from build123d import *

# Parameters (mm, degrees)
SKETCH_1_W          = 83
SKETCH_1_H          = 53
SKETCH_1_W_2        = 80.2
SKETCH_1_H_2        = 50.2
EXTRUDE_1_DEPTH     = 35
SKETCH_3_W          = 80.2
SKETCH_3_H          = 50.2
EXTRUDE_2_DEPTH     = 1.4
SKETCH_4_W          = 5
SKETCH_4_H          = 5
SKETCH_4_R          = 0.95
EXTRUDE_3_DEPTH     = 12
SKETCH_5_W          = 41
SKETCH_5_H          = 7
CUT_EXTRUDE_1_DEPTH = 10
SKETCH_6_W          = 10
SKETCH_6_H          = 7
SKETCH_6_H_2        = 9
SKETCH_6_W_2        = 10.2
SKETCH_6_H_3        = 6
CUT_EXTRUDE_2_DEPTH = 10
SKETCH_8_W          = 21
SKETCH_8_H          = 21
CUT_EXTRUDE_4_DEPTH = 10
SKETCH_9_W          = 13
SKETCH_9_H          = 9.6
CUT_EXTRUDE_5_DEPTH = 10
FILLET_1_R          = 1
FILLET_2_R          = 1
SKETCH_11_W         = 17.500857193
SKETCH_11_H         = 7
CUT_EXTRUDE_7_DEPTH = 10
FILLET_5_R          = 1
SKETCH_13_R         = 6
CUT_EXTRUDE_8_DEPTH = 10
FILLET_6_R          = 1
FILLET_7_R          = 1


with BuildPart() as part:
    # 草图1 → 凸台-拉伸1 (new body)
    with BuildSketch(Plane(origin=(0, 0, 0), x_dir=(1, 0, 0), z_dir=(0, 1, 0))):
        with Locations((40.1, 25.1)):
            Rectangle(SKETCH_1_W, SKETCH_1_H)
        with Locations((40.1, 25.1)):
            Rectangle(SKETCH_1_W_2, SKETCH_1_H_2, mode=Mode.SUBTRACT)
    extrude(amount=EXTRUDE_1_DEPTH)

    # 草图3 → 凸台-拉伸2 (add)
    with BuildSketch(Plane(origin=(0, 0, 0), x_dir=(1, 0, 0), z_dir=(0, 1, 0))):
        with Locations((40.1, 25.1)):
            Rectangle(SKETCH_3_W, SKETCH_3_H)
    extrude(amount=EXTRUDE_2_DEPTH)

    # 草图4 → 凸台-拉伸3 (add)
    # profile 1 of 4: a face of its own
    with BuildSketch(Plane(origin=(0, 1.4, 0), x_dir=(1, 0, 0), z_dir=(0, 1, 0))):
        with Locations((2.5, 47.7)):
            Rectangle(SKETCH_4_W, SKETCH_4_H)
        with Locations(Location((2.5, 47.7, 0), (0, 0, 270))):
            Circle(SKETCH_4_R, mode=Mode.SUBTRACT)
    # profile 2 of 4: a face of its own
    with BuildSketch(Plane(origin=(0, 1.4, 0), x_dir=(1, 0, 0), z_dir=(0, 1, 0))):
        with Locations((2.5, 2.5)):
            Rectangle(SKETCH_4_W, SKETCH_4_H)
        with Locations(Location((2.5, 2.5, 0), (0, 0, 270))):
            Circle(SKETCH_4_R, mode=Mode.SUBTRACT)
    # profile 3 of 4: a face of its own
    with BuildSketch(Plane(origin=(0, 1.4, 0), x_dir=(1, 0, 0), z_dir=(0, 1, 0))):
        with Locations((77.7, 47.7)):
            Rectangle(SKETCH_4_W, SKETCH_4_H)
        with Locations(Location((77.7, 47.7, 0), (0, 0, 270))):
            Circle(SKETCH_4_R, mode=Mode.SUBTRACT)
    # profile 4 of 4: a face of its own
    with BuildSketch(Plane(origin=(0, 1.4, 0), x_dir=(1, 0, 0), z_dir=(0, 1, 0))):
        with Locations((77.7, 2.5)):
            Rectangle(SKETCH_4_W, SKETCH_4_H)
        with Locations(Location((77.7, 2.184711345, 0), (0, 0, 270))):
            Circle(SKETCH_4_R, mode=Mode.SUBTRACT)
    extrude(amount=EXTRUDE_3_DEPTH)

    # 草图5 → 切除-拉伸1 (cut)
    with BuildSketch(Plane.ZY.offset(-80.2)):
        with Locations((-25.5, 17.9)):
            Rectangle(SKETCH_5_W, SKETCH_5_H)
    extrude(amount=-CUT_EXTRUDE_1_DEPTH, mode=Mode.SUBTRACT)

    # 草图6 → 切除-拉伸2 (cut)
    with BuildSketch(Plane(origin=(0, 0, 0), x_dir=(0, 0, -1), z_dir=(1, 0, 0))):
        with Locations((10, 17.9)):
            Rectangle(SKETCH_6_W, SKETCH_6_H)
        with Locations((40.2, 20.9)):
            Rectangle(SKETCH_6_W, SKETCH_6_H_2)
        with Locations((25.1, 18.4)):
            Rectangle(SKETCH_6_W_2, SKETCH_6_H_3)
    extrude(amount=-CUT_EXTRUDE_2_DEPTH, mode=Mode.SUBTRACT)

    # 草图8 → 切除-拉伸4 (cut)
    with BuildSketch(Plane.XY.offset(-50.2)):
        with Locations((64.7, 24.9)):
            Rectangle(SKETCH_8_W, SKETCH_8_H)
    extrude(amount=-CUT_EXTRUDE_4_DEPTH, mode=Mode.SUBTRACT)

    # 草图9 → 切除-拉伸5 (cut)
    with BuildSketch(Plane(origin=(0, 0, 0), x_dir=(-1, 0, 0), z_dir=(0, 0, -1))):
        with Locations((-40.1, 30.2)):
            Rectangle(SKETCH_9_W, SKETCH_9_H)
    extrude(amount=-CUT_EXTRUDE_5_DEPTH, mode=Mode.SUBTRACT)

    # 圆角1
    fillet_1_edges = [part.edges().sort_by_distance(p)[0] for p in [
        (80.9, 21.4, -5),
        (80.9, 14.4, -5),
        (80.9, 14.4, -46),
        (80.9, 21.4, -46),
        (-0.7, 14.4, -5),
        (-0.7, 21.4, -5),
        (-0.7, 21.4, -15),
        (-0.7, 14.4, -15),
        (-0.7, 25.4, -45.2),
        (-0.7, 16.4, -45.2),
        (-0.7, 16.4, -35.2),
        (-0.7, 25.4, -35.2),
        (-0.7, 15.4, -20),
        (-0.7, 21.4, -20),
        (-0.7, 15.4, -30.2),
        (75.2, 14.4, -50.9),
        (54.2, 14.4, -50.9),
        (46.6, 25.4, 0.7),
        (33.6, 25.4, 0.7),
        (5, 7.4, -5),
        (5, 7.4, -45.2),
        (75.2, 7.4, -45.2),
        (75.2, 7.4, -5),
    ]]
    fillet(fillet_1_edges, radius=FILLET_1_R)

    # 圆角2
    fillet_2_edges = [part.edges().sort_by_distance(p)[0] for p in [
        (40.1, 0, -51.6),
        (81.6, 0, -25.1),
        (40.1, 0, 1.4),
        (-1.4, 0, -25.1),
        (-1.4, 17.5, -51.6),
        (81.6, 17.5, -51.6),
        (81.6, 17.5, 1.4),
        (-1.4, 17.5, 1.4),
    ]]
    fillet(fillet_2_edges, radius=FILLET_2_R)

    # 草图11 → 切除-拉伸7 (cut)
    with BuildSketch(Plane(origin=(0, 0, 0), x_dir=(-1, 0, 0), z_dir=(0, 0, -1))):
        with Locations((-61.449571404, 17.9)):
            Rectangle(SKETCH_11_W, SKETCH_11_H)
    extrude(amount=-CUT_EXTRUDE_7_DEPTH, mode=Mode.SUBTRACT)

    # 圆角5
    fillet_5_edges = [part.edges().sort_by_distance(p)[0] for p in [
        (70.2, 14.4, 0.7),
        (70.2, 21.4, 0.7),
        (52.699142807, 21.4, 0.7),
        (52.699142807, 14.4, 0.7),
    ]]
    fillet(fillet_5_edges, radius=FILLET_5_R)

    # 草图13 → 切除-拉伸8 (cut)
    with BuildSketch(Plane(origin=(0, 0, 0), x_dir=(0, 0, -1), z_dir=(1, 0, 0))):
        with Locations((35.2, 7.4)):
            Circle(SKETCH_13_R)
    extrude(amount=-CUT_EXTRUDE_8_DEPTH, mode=Mode.SUBTRACT)

    # 圆角6
    fillet_6_edges = [part.edges().sort_by_distance(p)[0] for p in [
        (-0.7, 21.4, -30.2),
    ]]
    fillet(fillet_6_edges, radius=FILLET_6_R)

    # 圆角7
    fillet_7_edges = [part.edges().sort_by_distance(p)[0] for p in [
        (75.2, 35, -50.9),
        (54.2, 35, -50.9),
        (46.6, 35, 0.7),
        (33.6, 35, 0.7),
    ]]
    fillet(fillet_7_edges, radius=FILLET_7_R)


solid = part.part
Source: CAD feature listing. Evaluate the final solid. Frame: model axes, mm. A direction names the side the tool comes from. Coordinates: 2 decimals unless noted, no trailing zeros. Order: outer loops, then holes, each group sorted by start corner. A loop starts at its lowest first (then second) coordinate and runs counter-clockwise, first axis right, second up. Notation, with made-up numbers: M 65.25,31.25 L 83.25,31.25 A16 ccw 83.25,54.25 Z; hole C -16,61 d10. An arc over 180 degrees is marked long. Write each question's results on one line, items separated by ' | '. Start each with the question number.
1. Reachability of faces 4 (the face through (2.8, 7.3, -46.8)), 5 (the face through (-1, 35, -29)) from +Z, -Z, +X, -X, +Y, -Y: full face, straight path, thin tool, end or side. Return the list, or none.
2. Material intervals for L1, parallel to X at y = 5.5, z = -47.7; L2, parallel to X at y = 11, z = -15.5; L3, parallel to Z at x = 51, y = 4, sorted ascending.
3. Section B-B, the plane y = 7.4. State how many separate pieces and enclosed holes the cut face has, then the cut area to 3 significant figures.
4. Section C-C, the plane x = 67. Return the cut outline in (y, z).
5. Draft query along Y for faces 1 (the face through (80.2, 22, -25)), 2 (the face through (-0.69, 9.202, -40.923)), 3 (the face through (78, 1.4, -48)). Return one class per face: +Y half, -Y half, draft (parallel to the pull), parting line (faces both ways), or undercut.
6. Pin query (flat end, axial travel): pin 1 (0.7 mm diameter, centred on x = -1, y = 17, fed in from +Z); pin 2 (1.1 mm diameter, centred on x = 61, z = -51, fed in from +Y); pin 3 (0.6 mm diameter, centred on x = 78, z = -47.5, fed in from +Y). Return the tip coordinate at first contact, or that it passes through.
7. Section D-D, the plane z = -47.7. Return the cut outline in (x, y).
8. Section A-A, the plane z = -26.5. Return the cut outline in (x, y), then the cut area to 3 significant figures.
Solution:
1) face 4: +Y | face 5: +Z, -Z, +X, -X, +Y
2) L1: -1.4 to 1.55, 3.45 to 5, 75.2 to 76.75, 78.65 to 81.6 | L2: -1.4 to 0, 80.2 to 81.6 | L3: -51.6 to -50.2, 0 to 1.4
3) separate pieces: 1 | enclosed holes: 4 | area: 443 mm²
4) outline: M 0,-50.6 A1 ccw 1,-51.6 L 14.4,-51.6 L 14.4,-50.2 L 1.4,-50.2 L 1.4,0 L 14.4,0 L 14.4,1.4 L 1,1.4 A1 ccw 0,0.4 Z; M 21.4,0 L 35,0 L 35,1.4 L 21.4,1.4 Z
5) face 1: draft | face 2: undercut | face 3: +Y half
6) pin 1: z = 1.37 | pin 2: y = 14.4 | pin 3: y = 1.4
7) outline: M -1.4,1 A1 ccw -0.4,0 L 80.6,0 A1 ccw 81.6,1 L 81.6,35 L 80.2,35 L 80.2,13.4 L 78.65,13.4 L 78.65,1.4 L 76.75,1.4 L 76.75,13.4 L 75.2,13.4 L 75.2,1.4 L 5,1.4 L 5,13.4 L 3.45,13.4 L 3.45,1.4 L 1.55,1.4 L 1.55,13.4 L 0,13.4 L 0,35 L -1.4,35 Z
8) outline: M -1.4,1 A1 ccw -0.4,0 L 80.6,0 A1 ccw 81.6,1 L 81.6,14.4 L 80.2,14.4 L 80.2,1.4 L 0,1.4 L 0,15.4 L -1.4,15.4 Z; M -1.4,21.4 L 0,21.4 L 0,35 L -1.4,35 Z; M 80.2,21.4 L 81.6,21.4 L 81.6,35 L 80.2,35 Z | area: 192 mm²
